Source: three-view drawing plus pictorial views. Frame: mm from the lowest corner of the part. A direction names the side the tool comes from. Give positions to 0.01 mm unless a question says otherwise; leave off trailing zeros. Order: outer loops, then holes, each group sorted by start corner. A loop starts at its lowest first (then second) coordinate and runs counter-clockwise, first axis right, second up. Notation, with made-up numbers: (49, 44.5) -> (94, 44.5) arc R18 ccw to (94, 65.5) -> close; hole circle Ø9 at (68, -6.75). An arc over 180 degrees is marked (long way). One line per question, with ' | ' between items.
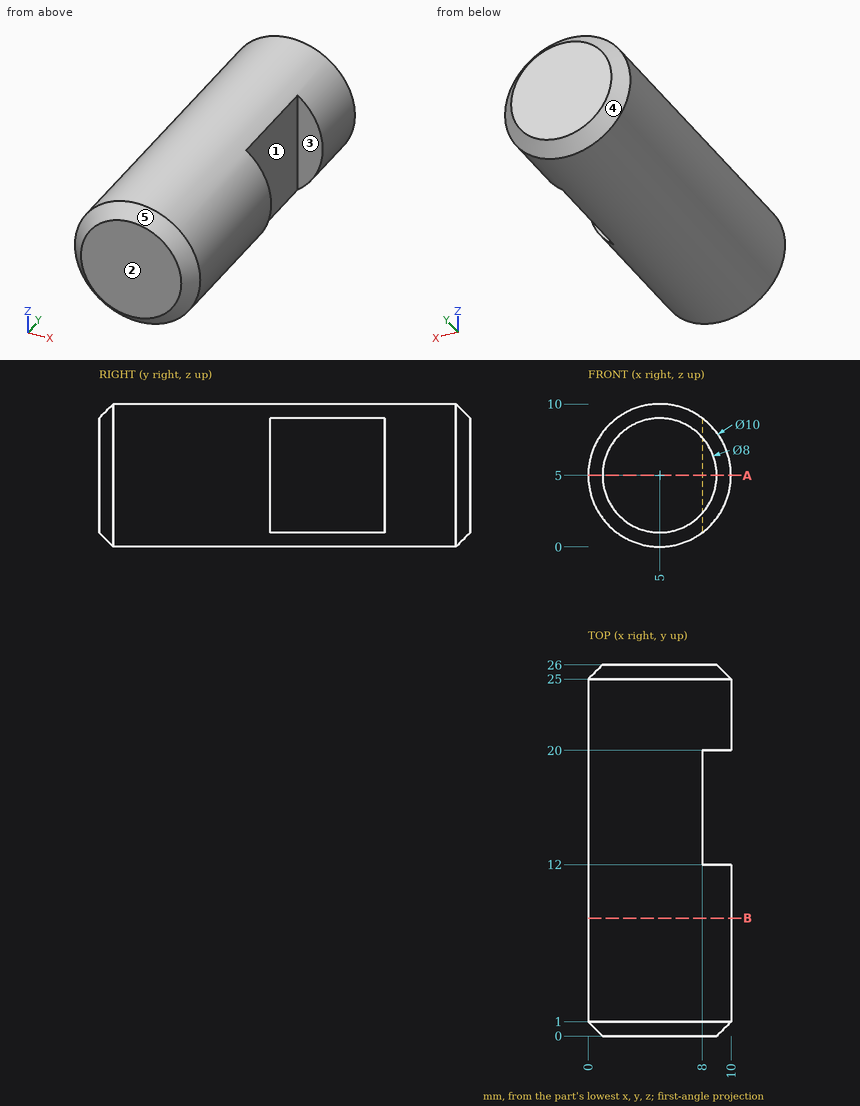
1) Pull-direction query (Y, two-part tool) for the marked faces 3, 4 and 5; classes: +Y half, -Y half, draft (parallel to the pull), parting line (faces both ways), or undercut.
Check result:
face 3: undercut | face 4: +Y half | face 5: -Y half
2) Section A-A on z = 5. Return loops of the section in (x, y), plus the area to 3 significant figures.
Check result:
outline: (0, 1) -> (1, 0) -> (9, 0) -> (10, 1) -> (10, 12) -> (8, 12) -> (8, 20) -> (10, 20) -> (10, 25) -> (9, 26) -> (1, 26) -> (0, 25) -> close | area: 242 mm^2
3) Contact query for flat-ended pins moving along their axis: pin 1 Ø3 at (x, y) = (8.5, 21) entering from -Z; pin 2 Ø1 at (x, y) = (6.5, 6) entering from +Z; pin 3 Ø6 at (x, y) = (4, 20) entering from -Z; pin 4 Ø1 at (y, z) = (14.5, 7) entering from +X. Output: stop coordinate, or through.
Check result:
pin 1: stops at z = 0.42 | pin 2: stops at z = 9.9 | pin 3: stops at z = 0 | pin 4: stops at x = 8
4) Set-up query: the marked faces 1 and 2. Return all of +Z, -Z, +X, -X, +Y, -Y with unobstructed straight access to the full face (end or side cutting, diameter ignored); none if empty.
Check result:
face 1: +Z, -Z, +X | face 2: +Z, -Z, +X, -X, -Y
5) Section B-B on y = 8.25. Return loops of the section in (x, z), plus the area to 3 significant figures.
Check result:
outline: circle Ø10 at (5, 5) | area: 78.5 mm^2
6) Material intervals for probe 1 along Y at (x, z) = (8.5, 4); probe 2 along Y at (x, z) = (9, 6); probe 3 along Z at (x, y) = (2, 8), sorted ascending. Write a range as from..to.
Check result:
probe 1: y = 0..12, 20..26 | probe 2: y = 0.12..12, 20..25.88 | probe 3: z = 1..9
